Can you work these out from the model? Positions are in its coordinate system, mm. A direction names the side the tool comes from. Give positions to 0.01 mm unless a question says otherwise; leave off trailing zeros. Loops run counter-clockwise (first coordinate to the right, second up) from the corner with the lowest first, then second, coordinate; pieces in that order, holes last. Notation, with made-up numbers: (24, 77.25) -> (64, 77.25) arc R24 cw to (64, 102.25) -> close; hole circle Ø1 at (-21, -18.75). An arc over 180 degrees is marked (long way). Return JSON: item names as keys, results as strings. Group by question number.
Q1. Will these pins go through, and if not, where does the flat tip stop? pin 1 (6.5 mm diameter, centred on y = 13, z = 5.5, fed in from -X); pin 2 (2.5 mm diameter, centred on x = 6, y = 3, fed in from -Z); pin 3 (2.5 mm diameter, centred on y = -8.5, z = 3, fed in from +X).
Q2. Suppose I cut it at C-C, the plane x = 3. Please give me the cut outline in (y, z).
Q3. Suppose I cut it at A-A, the plane y = 17.5. Please give me the cut outline in (x, z), and give its area (3 significant figures).
Q4. Suppose I cut it at D-D, the plane z = -12. Please give me the cut outline in (x, y), and give its area (3 significant figures).
Q5. Thinking about a two-plate mould opening in Y: for faces 1 (the cylindrical face through (-17.04, 18.39, -8.38)), 2 (the flat face through (-7, -8, 12)), 3 (the flat face through (-2, 0, -8)), which applies, pulls with the +Y half, pulls with the -Y half, needs draft (parallel to the pull), parting line crosses it, or undercut?
Q6. Which directions (+Z, -Z, +X, -X, +Y, -Y) give clear straight access to the entire face, cutting with the end or side of a thin tool? Please do faces 4 (the flat face through (-2, 2, 5)), 5 (the flat face through (-3, -9, 0)), 6 (the flat face through (8, 2, 0)), 7 (the flat face through (8, 0, 3)).
Q7. I need wall thicknesses on line 1 along X through (y, z) = (8, 12); line 2 along Z through (x, y) = (-1, 4); line 3 along Z through (x, y) = (12.75, 17.5). Which ranges of each line are inside material? Lowest first, please. Write a range as [from, to].
```python
from build123d import *

# Parameters (mm, degrees)
F0_R     = 1
F1_DEPTH = 17
F2_W     = 5
F2_H     = 5
F3_DEPTH = 5
F4_R     = 1
F5_DEPTH = 17
F6_R     = 1
F7_DEPTH = 17


with BuildPart() as f1:
    # F0 (on Front) → F1 (new body)
    with BuildSketch(Plane.XZ):
        with BuildLine():
            Line((-5, 0), (0, 0))
            Line((0, 0), (0, 5))
            Line((0, 5), (-15, 20))
            ThreePointArc((-15, 20), (-20, 20), (-20, 15))
            Line((-20, 15), (-5, 0))
        make_face()
        with Locations((-17.5, 17.5)):
            Circle(F0_R, mode=Mode.SUBTRACT)
    extrude(amount=F1_DEPTH)

    # F2 (on face) → F3 (join)
    with BuildSketch(Plane(origin=(0, 0, 0), x_dir=(-1, 0, 0), z_dir=(0, 1, 0))):
        with Locations((2.5, 2.5)):
            Rectangle(F2_W, F2_H)
    extrude(amount=F3_DEPTH)

    # F4 (on face) → F5 (join)
    with BuildSketch(Plane.YZ):
        with BuildLine():
            Line((0, 5), (0, 0))
            Line((0, 0), (5, 0))
            Line((5, 0), (20, 15))
            ThreePointArc((20, 15), (20, 20), (15, 20))
            Line((15, 20), (0, 5))
        make_face()
        with Locations((17.5, 17.5)):
            Circle(F4_R, mode=Mode.SUBTRACT)
    extrude(amount=F5_DEPTH)

    # F6 (on face) → F7 (join)
    with BuildSketch(Plane(origin=(0, 0, 0), x_dir=(1, 0, 0), z_dir=(0, 0, -1))):
        with BuildLine():
            Line((0, -5), (0, 0))
            Line((0, 0), (-5, 0))
            Line((-5, 0), (-20, -15))
            ThreePointArc((-20, -15), (-20, -20), (-15, -20))
            Line((-15, -20), (0, -5))
        make_face()
        with Locations((-17.5, -17.5)):
            Circle(F6_R, mode=Mode.SUBTRACT)
    extrude(amount=F7_DEPTH)


solid = f1.part
```
Ans:
{
 "1": {"pin 1": "stops at x = 0", "pin 2": "stops at z = 0", "pin 3": "stops at x = 0"},
 "2": {"outline": "(0, 0) -> (5, 0) -> (20, 15) arc R3.54 ccw to (15, 20) -> (0, 5) -> close; hole circle Ø2 at (17.5, 17.5)"},
 "3": {"outline": "(-21.04, -17) -> (-18.5, -17) -> (-18.5, 0) -> (-21.04, 0) -> close; (-16.5, -17) -> (-12.5, -17) -> (-12.5, 0) -> (-16.5, 0) -> close; (0, 12.5) -> (17, 12.5) -> (17, 16.5) -> (0, 16.5) -> close; (0, 18.5) -> (17, 18.5) -> (17, 21.04) -> (0, 21.04) -> close", "area": "222 mm^2"},
 "4": {"outline": "(-20, 15) -> (-5, 0) -> (0, 0) -> (0, 5) -> (-15, 20) arc R3.54 ccw to start; hole circle Ø2 at (-17.5, 17.5)", "area": "179 mm^2"},
 "5": {"face 1": "undercut", "face 2": "needs draft", "face 3": "pulls with the -Y half"},
 "6": {"face 4": "+Z, -X, +Y", "face 5": "-Z, +X, -X, -Y", "face 6": "-Z, +X, +Y, -Y", "face 7": "+Z, -Z, +X, -Y"},
 "7": {"line 1": "x = [0, 17]", "line 2": "z = [-17, 5]", "line 3": "z = [12.5, 16.5], [18.5, 21.04]"}
}
